Source: CAD feature listing. Evaluate the final solid. Frame: model axes, mm. Face numbers are marked on the shaded views. A direction names the side the tool comes from. Give positions to 0.01 mm unless a question says otherwise; leave off trailing zeros. Write each loop counter-clockwise with the first axis right and the second up, starting at its lowest first coordinate (ties: lowest second). Pieces come first, ordered by that corner, then holes. Notation, with made-up numbers: (77, 87.25) -> (82, 87.25) arc R17 cw to (82, 93.25) -> close; hole circle Ø3 at (-7, 9.25). An arc over 180 degrees is marked (long way). Write item = value, one per line.
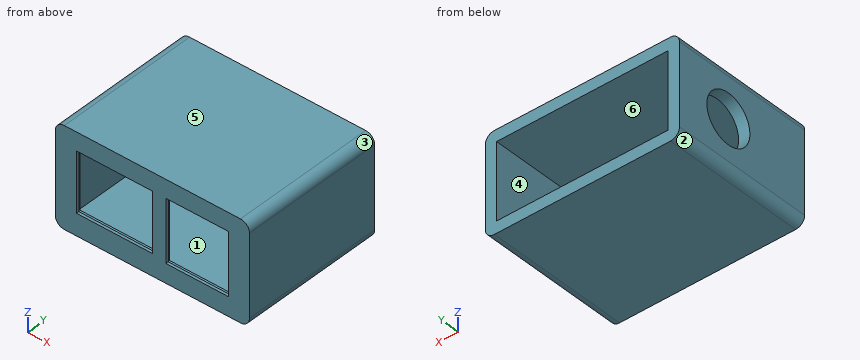
from build123d import *

# Parameters (mm, degrees)
BOSS_EXTRUDE1_DEPTH = 2
SKETCH2_W           = 18.8
SKETCH2_H           = 15.2
SKETCH2_W_2         = 15.8
SKETCH2_H_2         = 15.8
CUT_EXTRUDE1_DEPTH  = 1.4
SKETCH3_W           = 16.8
SKETCH3_H           = 13.2
SKETCH3_W_2         = 13.8
SKETCH3_H_2         = 13.8
CUT_EXTRUDE2_DEPTH  = 25.191114071
BOSS_EXTRUDE3_DEPTH = 30
FILLET1_R           = 10
SKETCH15_W          = 38
SKETCH15_H          = 16.8
CUT_EXTRUDE3_DEPTH  = 39.512984823
CUT_EXTRUDE4_REACH  = 56.717
SKETCH16_R          = 5.5


with BuildPart() as part:
    # Sketch1 → Boss-Extrude1 (new body)
    with BuildSketch(Plane(origin=(0, 0, 0), x_dir=(1, 0, 0), z_dir=(0, 1, 0))):
        with BuildLine():
            Line((19.5, -11), (-19.5, -11))
            ThreePointArc((-19.5, -11), (-20.914213562, -10.414213562), (-21.5, -9))
            Line((-21.5, -9), (-21.5, 9))
            ThreePointArc((-21.5, 9), (-20.914213562, 10.414213562), (-19.5, 11))
            Line((-19.5, 11), (19.5, 11))
            ThreePointArc((19.5, 11), (20.914213562, 10.414213562), (21.5, 9))
            Line((21.5, 9), (21.5, -9))
            ThreePointArc((21.5, -9), (20.914213562, -10.414213562), (19.5, -11))
        make_face()
    extrude(amount=BOSS_EXTRUDE1_DEPTH)

    # Sketch2 → Cut-Extrude1 (cut)
    with BuildSketch(Plane(origin=(0, 2, 0), x_dir=(1, 0, 0), z_dir=(0, 1, 0))):
        with Locations((-8.4, -0.4)):
            Rectangle(SKETCH2_W, SKETCH2_H)
        with Locations((9.9, -0.1)):
            Rectangle(SKETCH2_W_2, SKETCH2_H_2)
    extrude(amount=-CUT_EXTRUDE1_DEPTH, mode=Mode.SUBTRACT)

    # Sketch3 → Cut-Extrude2 (cut, through all)
    with BuildSketch(Plane(origin=(0, 0.6, 0), x_dir=(1, 0, 0), z_dir=(0, 1, 0))):
        with Locations((-8.4, -0.4)):
            Rectangle(SKETCH3_W, SKETCH3_H)
        with Locations((9.9, -0.1)):
            Rectangle(SKETCH3_W_2, SKETCH3_H_2)
    extrude(amount=-CUT_EXTRUDE2_DEPTH, mode=Mode.SUBTRACT)

    # Sketch13 → Boss-Extrude3 (add)
    with BuildSketch(Plane(origin=(0, 2, 0), x_dir=(1, 0, 0), z_dir=(0, 1, 0))):
        with BuildLine():
            ThreePointArc((-21.5, -9), (-20.914213562, -10.414213562), (-19.5, -11))
            Line((-19.5, -11), (19.5, -11))
            ThreePointArc((19.5, -11), (20.914213562, -10.414213562), (21.5, -9))
            Line((21.5, -9), (21.5, 9))
            ThreePointArc((21.5, 9), (20.914213562, 10.414213562), (19.5, 11))
            Line((19.5, 11), (-19.5, 11))
            ThreePointArc((-19.5, 11), (-20.914213562, 10.414213562), (-21.5, 9))
            Line((-21.5, 9), (-21.5, -9))
        make_face()
        with BuildLine():
            ThreePointArc((17.5, 8), (18.207106781, 7.707106781), (18.5, 7))
            Line((18.5, 7), (18.5, -7))
            ThreePointArc((18.5, -7), (18.306225775, -7.591607978), (17.8, -7.953939201))
            Line((17.8, -7.953939201), (17.8, -8))
            Line((17.8, -8), (-17.8, -8))
            Line((-17.8, -8), (-17.8, -7.953939201))
            ThreePointArc((-17.8, -7.953939201), (-18.306225775, -7.591607978), (-18.5, -7))
            Line((-18.5, -7), (-18.5, 7))
            ThreePointArc((-18.5, 7), (-18.207106781, 7.707106781), (-17.5, 8))
            Line((-17.5, 8), (17.5, 8))
        make_face(mode=Mode.SUBTRACT)
    extrude(amount=BOSS_EXTRUDE3_DEPTH)

    # Fillet1
    # the kernel refuses this fillet: 10 mm, written as the material it takes off along each edge
    with BuildSketch(Plane(origin=(17.8, 2, 7.953939201), x_dir=(0.906100611464274, 0, -0.42306226717123885), z_dir=(0, 1, 0))) as fillet1_piece_1:
        with BuildLine():
            CenterArc((1.580945974, -9.912835739), FILLET1_R, 97.570469618, 1.638937345)
            Line((-0.019486586, -0.041735718), (0, 0))
            ThreePointArc((0, 0), (0.131745498, -0.008716426), (0.263490996, 0))
        make_face()
    extrude(amount=30.658727489, mode=Mode.SUBTRACT)

    # Sketch15 → Cut-Extrude3 (cut, through all)
    with BuildSketch(Plane(origin=(0, 2, 0), x_dir=(1, 0, 0), z_dir=(0, 1, 0))):
        Rectangle(SKETCH15_W, SKETCH15_H)
    extrude(amount=CUT_EXTRUDE3_DEPTH, mode=Mode.SUBTRACT)

    # Sketch16 → Cut-Extrude4 (cut, up to next)
    with BuildSketch(Plane.ZY.offset(21.5), mode=Mode.PRIVATE) as cut_extrude4_sk1:
        with Locations((0, 19.5)):
            Circle(SKETCH16_R)
    cut_extrude4_tool1 = extrude(cut_extrude4_sk1.sketch, amount=-CUT_EXTRUDE4_REACH, mode=Mode.PRIVATE) & part.part
    add(cut_extrude4_tool1.solids().sort_by_distance((-21.5, 19.5, 0))[0], mode=Mode.SUBTRACT)


solid = part.part
(1) Pull-direction query (Z, two-part tool) for the marked faces 1, 2, 3 and 4; classes: pulls with the +Z half, pulls with the -Z half, needs draft (parallel to the pull), parting line crosses it, or undercut.
Values follow:
face_1 = undercut
face_2 = pulls with the -Z half
face_3 = pulls with the +Z half
face_4 = undercut
(2) Section query D-D (y = 19.5). Return loops of the section in (x, z).
Values follow:
outline = (-21.5, -9) arc R2 ccw to (-19.5, -11) -> (19.5, -11) arc R2 ccw to (21.5, -9) -> (21.5, 9) arc R2 ccw to (19.5, 11) -> (-19.5, 11) arc R2 ccw to (-21.5, 9) -> (-21.5, 5.5) -> (-19, 5.5) -> (-19, 8.4) -> (19, 8.4) -> (19, -8.4) -> (-19, -8.4) -> (-19, -5.5) -> (-21.5, -5.5) -> close
(3) Access query for the marked faces 5 and 6. Directions: +Z, -Z, +X, -X, +Y, -Y. A direction counts if a zero-diameter tool reaches every point of the face in a straight line with its end or side. Return the directions, or none.
Values follow:
face_5 = +Z, +X, -X, +Y, -Y
face_6 = +Y
(4) Section query C-C (y = 4.5). Return loops of the section in (x, z), plus the area to 3 significant figures.
Values follow:
outline = (-21.5, -9) arc R2 ccw to (-19.5, -11) -> (19.5, -11) arc R2 ccw to (21.5, -9) -> (21.5, 9) arc R2 ccw to (19.5, 11) -> (-19.5, 11) arc R2 ccw to (-21.5, 9) -> close; hole (-19, -8.4) -> (19, -8.4) -> (19, 8.4) -> (-19, 8.4) -> close
area = 304 mm2
(5) Section query B-B (x = -1). Return loops of the section in (y, z).
Values follow:
outline = (0, -11) -> (32, -11) -> (32, -8.4) -> (2, -8.4) -> (2, -7.2) -> (0.6, -7.2) -> (0.6, -6.2) -> (0, -6.2) -> close; (0, 7) -> (0.6, 7) -> (0.6, 8) -> (2, 8) -> (2, 8.4) -> (32, 8.4) -> (32, 11) -> (0, 11) -> close
(6) Section query A-A (z = 0). Return loops of the section in (x, y), plus the area to 3 significant figures.
Values follow:
outline = (-21.5, 0) -> (-16.8, 0) -> (-16.8, 0.6) -> (-17.8, 0.6) -> (-17.8, 2) -> (-19, 2) -> (-19, 14) -> (-21.5, 14) -> close; (-21.5, 25) -> (-19, 25) -> (-19, 32) -> (-21.5, 32) -> close; (0, 0) -> (3, 0) -> (3, 0.6) -> (2, 0.6) -> (2, 2) -> (1, 2) -> (1, 0.6) -> (0, 0.6) -> close; (16.8, 0) -> (21.5, 0) -> (21.5, 32) -> (19, 32) -> (19, 2) -> (17.8, 2) -> (17.8, 0.6) -> (16.8, 0.6) -> close
area = 142 mm2
(7) Material intervals for line 1 (X direction, y = 17, z = 8.25); line 2 (Z direction, x = 11, y = 17); line 3 (Y direction, x = -20.85, z = 0), sorted ascending.
Values follow:
line_1 = -21.5 to -19, 19 to 21.5
line_2 = -11 to -8.4, 8.4 to 11
line_3 = 0 to 14, 25 to 32
